Part model, mm, in its own coordinate system. A direction names the side the tool comes from. Coordinates: 2 decimals unless noted, no trailing zeros. Loops run counter-clockwise (first coordinate to the right, second up) from the corner with the lowest first, then second, coordinate; pieces in that order, holes last. Notation, with made-up numbers: M 83.5,15 L 92.5,15 A18 cw 92.5,48 Z; hole C 84,2.5 d2. An arc over 180 degrees is marked long. Answer as a JSON object with one key per item and string values. Group by question number.
1. Saw through at A-A on y = 54. Write the cut outline in (x, z).
2. Saw through at D-D on z = 19. Write the cut outline in (x, y), then the cut area to 3 significant figures.
3. Drill centre lines: L1, parallel to X at y = 24, z = -3.5; L2, parallel to Y at x = -40, z = -21; L3, parallel to Y at x = -4.5, z = 2. Where is each one in solid material? Low to high.
4. Mould opens along X. For faces 6 (the face through (20, 22, 34)), 7 (the face through (0, 17, 28)), 8 (the face through (40, 23, 40)), 9 (the face through (-60, 6, 1)) say: released by +X, released by -X, zero draft, split by the parting line, or undercut.
5. Saw through at C-C on y = 5. Write the cut outline in (x, z).
6. Drop flat-ended pins along their axis: pin 1 Ø6 at (x, y) = (-34, 29.5) entering from +Z; pin 2 Ø9 at (x, z) = (-12.5, 4.5) entering from +Y; pin 3 Ø1 at (x, z) = (-45, 14.5) entering from -Y; pin 4 Ø20 at (x, z) = (45.5, -2) entering from +Y. Give the stop position or say it passes through.
7. Saw through at B-B on x = 53.5. Write the cut outline in (y, z).
8. 3-axis set-ups, long thin cutter, end or side, ignore diameter. For faces 1 (the face through (-40, 30, 0)), 2 (the face through (-20, 14, 34)), 3 (the face through (42, 46, 0)), 4 (the face through (-26, 34, -15)), 5 (the face through (-26, 34, 15)): which of +Z, -Z, +X, -X, +Y, -Y reach the whole face in a straight line?
from build123d import *

# Parameters (mm, degrees)
BOSS_EXTRUDE1_DEPTH = 60
CUT_EXTRUDE2_DEPTH  = 40
SKETCH8_W           = 100
SKETCH8_H           = 30
BOSS_EXTRUDE2_DEPTH = 40
SKETCH9_W           = 25
SKETCH9_H           = 14
CUT_EXTRUDE3_DEPTH  = 94.808315196


with BuildPart() as part:
    # Sketch1 → Boss-Extrude1 (new body)
    with BuildSketch(Plane(origin=(0, 0, 0), x_dir=(1, 0, 0), z_dir=(0, 1, 0))):
        Polygon((-20, -28), (-20, -40), (-60, -40), (-60, 40), (60, 40), (60, -40), (20, -40), (20, -28), align=None)
    extrude(amount=BOSS_EXTRUDE1_DEPTH)

    # Sketch7 → Cut-Extrude2 (cut, symmetric)
    with BuildSketch(Plane.XY):
        Polygon((60, 60), (-60, 12), (-60, 60), align=None)
    extrude(amount=CUT_EXTRUDE2_DEPTH, both=True, mode=Mode.SUBTRACT)

    # Sketch8 → Boss-Extrude2 (add)
    with BuildSketch(Plane(origin=(0, 0, 0), x_dir=(1, 0, 0), z_dir=(0, 1, 0))):
        with Locations((10, 0)):
            Rectangle(SKETCH8_W, SKETCH8_H)
    extrude(amount=BOSS_EXTRUDE2_DEPTH)

    # Sketch9 → Cut-Extrude3 (cut, through all)
    with BuildSketch(Plane(origin=(0, 0, 0), x_dir=(0, 0, -1), z_dir=(1, 0, 0))):
        with Locations((0, 53)):
            Rectangle(SKETCH9_W, SKETCH9_H)
    extrude(amount=CUT_EXTRUDE3_DEPTH, mode=Mode.SUBTRACT)


solid = part.part
Outcome:
{
 "1": {"outline": "M 45,-40 L 60,-40 L 60,-12.5 L 45,-12.5 Z; M 45,12.5 L 60,12.5 L 60,40 L 45,40 Z"},
 "2": {"outline": "M -60,0 L 60,0 L 60,60 L -60,12 Z", "area": "4,320 mm²"},
 "3": {"L1": "x = -40 to 60", "L2": "y = 0 to 20", "L3": "y = 0 to 40"},
 "4": {"face 6": "undercut", "face 7": "undercut", "face 8": "zero draft", "face 9": "released by -X"},
 "5": {"outline": "M -60,-40 L 60,-40 L 60,40 L 20,40 L 20,28 L -20,28 L -20,40 L -60,40 Z"},
 "6": {"pin 1": "stops at z = 15", "pin 2": "stops at y = 40", "pin 3": "stops at y = 0", "pin 4": "stops at y = 46"},
 "7": {"outline": "M 0,-40 L 57.4,-40 L 57.4,-12.5 L 46,-12.5 L 46,12.5 L 57.4,12.5 L 57.4,40 L 0,40 Z"},
 "8": {"face 1": "+Z, -Z, -X, +Y", "face 2": "+Z, +Y, -Y", "face 3": "+X, -X, +Y", "face 4": "-Z, -X, +Y", "face 5": "+Z, -X, +Y"}
}
